Could you check a few things on this drawing? It's one solid part, dimensions in mm from its lowest x, y, z. A direction names the side the tool comes from. Round coordinates to 2 decimals unless told otherwise and drop trailing zeros. Order: outer loops, then holes, each group sorted by start corner. A loop starts at its lowest first (then second) coordinate and runs counter-clockwise, first axis right, second up.
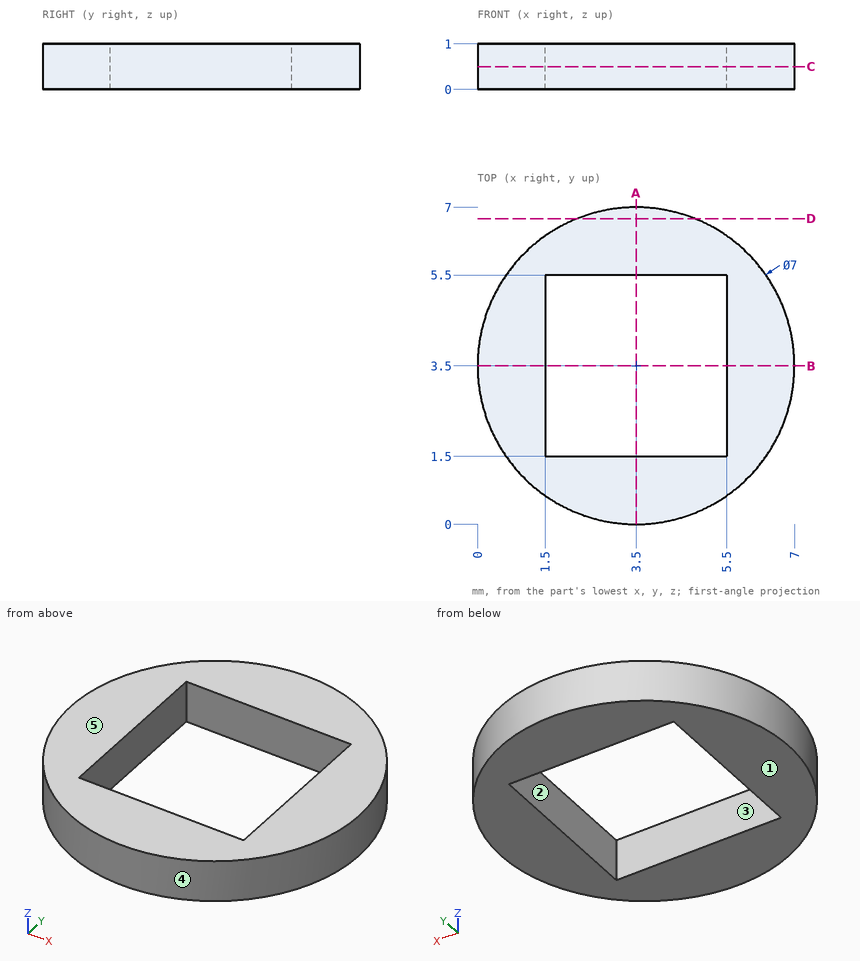
(1) I'm going to push a flat-ended pin straight in: pin 1 Ø0.5 at (y, z) = (4.5, 0.5) entering from -X. Where does the tip first touch, or does it pass through?
(2) I want a section at C-C, the plane z = 0.5. List the corners of the cut face in (x, y) for me.
(3) On a 3-axis mill with a long thin cutter (end or side, diameter ignored), from which of +Z, -Z, +X, -X, +Y, -Y can I reach the whole of each face in a straight line? I mean the marked faces 1 and 2. Say none if no direction works.
(4) I want a section at A-A, the plane x = 3.5. List the corners of the cut face in (y, z) for me, plus the area to 3 significant figures.
(5) Please list where these lines run through material, in increasing order: probe 1 along Y at (x, z) = (4, 0.55); probe 2 along X at (y, z) = (2.5, 0.2); probe 3 along Y at (x, z) = (5, 0.9).
(6) I want a section at D-D, the plane y = 6.75. List the corners of the cut face in (x, z) for me, plus the area to 3 significant figures.
(7) If we mould it in two halves opening along X, with no side actions, what happens to the marked faces 3, 4 and 5? For each: pulls with the +X half, pulls with the -X half, needs draft (parallel to the pull), parting line crosses it, or undercut.
Ans:
1. pin 1: stops at x = 0.08
2. outline: circle Ø7 at (3.5, 3.5); hole (1.5, 1.5) - (5.5, 1.5) - (5.5, 5.5) - (1.5, 5.5) - close
3. face 1: -Z, +X, -X, +Y, -Y
3. face 2: +Z, -Z
4. outline: (0, 0) - (1.5, 0) - (1.5, 1) - (0, 1) - close; (5.5, 0) - (7, 0) - (7, 1) - (5.5, 1) - close
4. area: 3.00 mm2
5. probe 1: y = 0.04 to 1.5, 5.5 to 6.96
5. probe 2: x = 0.15 to 1.5, 5.5 to 6.85
5. probe 3: y = 0.34 to 1.5, 5.5 to 6.66
6. outline: (2.2, 0) - (4.8, 0) - (4.8, 1) - (2.2, 1) - close
6. area: 2.60 mm2
7. face 3: undercut
7. face 4: parting line crosses it
7. face 5: needs draft
